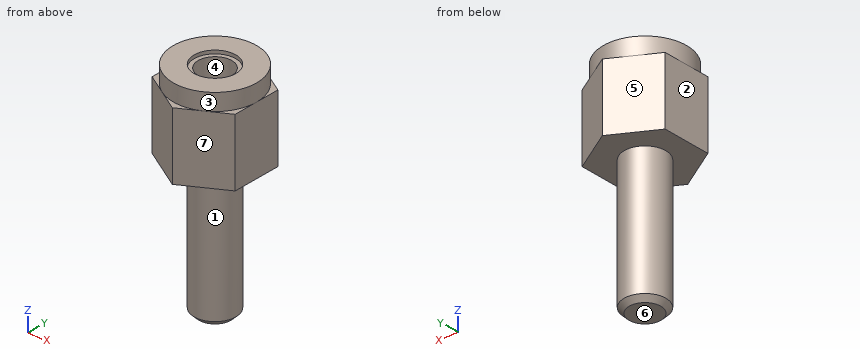
Autodesk Inventor part; units mm, degrees
ref_plane "YZ Plane" through (0, 0, 0) normal (1, 0, 0) x (0, 1, 0)
ref_plane "XZ Plane" through (0, 0, 0) normal (0, 1, 0) x (-1, 0, 0)
ref_plane "XY Plane" through (0, 0, 0) normal (0, 0, 1) x (1, 0, 0)
sketch "Skizze1" plane through (0, 0, 0) normal (0, 0, 1) x (1, 0, 0)
  line L0 (0, 2.8868) -> (2.5, 1.4434)
  line L1 (2.5, 1.4434) -> (2.5, -1.4434)
  line L2 (2.5, -1.4434) -> (0, -2.8868)
  line L3 (0, -2.8868) -> (-2.5, -1.4434)
  line L4 (-2.5, -1.4434) -> (-2.5, 1.4434)
  line L5 (-2.5, 1.4434) -> (0, 2.8868)
  point P0 (0, 0)
  point P1 (0, 0)
  dimension "d0" = 5
extrude "Extrusion1" add sketch "Skizze1" along normal blind 4
sketch "Skizze2" plane through (0, 0, 4) normal (0, 0, 1) x (1, 0, 0)
  circle A0 centre (0, 0) radius 2.5
  line L0 (2.5, -1.4434) -> (2.5, 1.4434)
extrude "Extrusion2" add sketch "Skizze2" along normal blind 1
sketch "Skizze3" plane through (0, 0, 0) normal (0, 0, -1) x (-1, 0, 0)
  circle A0 centre (0, 0) radius 1.25
  dimension "d6" = 2.5
extrude "Extrusion3" add sketch "Skizze3" along normal blind 8
thread "Gewinde1"
chamfer "Fase1" distance 0.3 angle 45 1 edges at (1.25, 0, -8)
sketch "Skizze4" plane through (0, 0, 5) normal (0, 0, 1) x (1, 0, 0)
  point P0 (0, 0)
  point P1 (0, 0)
hole "Bohrung1" at (0, 0, 5) direction (0, 0, -1) diameter 2.013 depth 4.5 tip angle 118 counterbore diameter 2.5 counterbore depth 0.2
properties part number "distanzhalter_schraube"
Could you check a few things on this model? Use its own coordinates, in mm. Face numbers are marked on the shaded views. A direction names the side the tool comes from. Coordinates: 2 decimals unless noted, no trailing zeros. Write each loop counter-clockwise with the first axis right and the second up, starting at its lowest first coordinate (ties: lowest second). Pieces come first, ordered by that corner, then holes. Notation, with made-up numbers: (19.25, 40.25) - (24.25, 40.25) arc R24 ccw to (24.25, 63.25) - close; hole circle Ø11 at (7.5, -16.5). An arc over 180 degrees is marked (long way). Use a Markdown table: item, result.
Q1. Imagine slicing it at C-C (x = 2.2). List the corners of the cut face in (y, z) for me, and give its area (3 significant figures).
Geometry check:
| item | result |
|---|---|
| outline | (-1.62, 0) - (1.62, 0) - (1.62, 4) - (1.19, 4) - (1.19, 5) - (-1.19, 5) - (-1.19, 4) - (-1.62, 4) - close |
| area | 15.3 mm2 |
Q2. Imagine slicing it at A-A (z = 0.25). List the corners of the cut face in (x, y) for me.
Geometry check:
| item | result |
|---|---|
| outline | (-2.5, -1.44) - (0, -2.89) - (2.5, -1.44) - (2.5, 1.44) - (0, 2.89) - (-2.5, 1.44) - close; hole circle Ø1.18 at (0, 0) |
Q3. Imagine slicing it at D-D (z = -1.5). List the corners of the cut face in (x, y) for me, and give its area (3 significant figures).
Geometry check:
| item | result |
|---|---|
| outline | circle Ø2.5 at (0, 0) |
| area | 4.91 mm2 |
Q4. I'm going to push flat-ended pins straight in: pin 1 Ø3 at (y, z) = (-2, -5) entering from -X; pin 2 Ø1.5 at (y, z) = (1.5, -4) entering from -X; pin 3 Ø3 at (x, z) = (-1, -2) entering from -Y. Where does each tip first touch, or does it pass through?
Geometry check:
| item | result |
|---|---|
| pin 1 | stops at x = -1.15 |
| pin 2 | stops at x = -1 |
| pin 3 | stops at y = -1.25 |
Q5. Please list where these lines run through material, in increasing order: L1, parallel to X at y = 0, z = 3.6; L2, parallel to Z at x = 0.1, y = -1.5; L3, parallel to X at y = 0, z = 4.9.
Geometry check:
| item | result |
|---|---|
| L1 | x = -2.5 to -1.01, 1.01 to 2.5 |
| L2 | z = 0 to 5 |
| L3 | x = -2.5 to -1.25, 1.25 to 2.5 |
Q6. Which directions (+Z, -Z, +X, -X, +Y, -Y) give clear straight access to the entire face, cutting with the end or side of a thin tool? Please do the marked faces 1, 2 and 3.
Geometry check:
| item | result |
|---|---|
| face 1 | -Z |
| face 2 | +Z, -Z, -X, +Y, -Y |
| face 3 | +Z |
Q7. Thinking about a two-plate mould opening in X: for the marked faces 4, 5, 6 and 7, which applies, +X half, -X half, draft (parallel to the pull), parting line (faces both ways), or undercut?
Geometry check:
| item | result |
|---|---|
| face 4 | undercut |
| face 5 | -X half |
| face 6 | draft |
| face 7 | +X half |
Q8. Imagine slicing it at B-B (y = 1.85). List the corners of the cut face in (x, z) for me.
Geometry check:
| item | result |
|---|---|
| outline | (-1.8, 0) - (1.8, 0) - (1.8, 4) - (1.68, 4) - (1.68, 5) - (-1.68, 5) - (-1.68, 4) - (-1.8, 4) - close |
